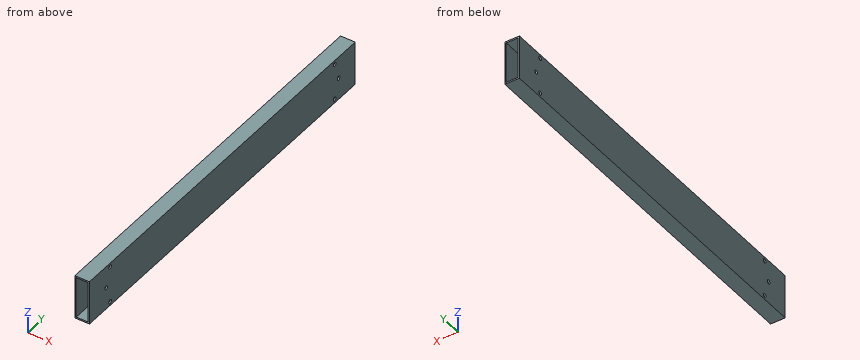
```python
from build123d import *

# Parameters (mm, degrees)
F0_W     = 30
F0_H     = 90
F1_DEPTH = 400
F2_T     = -3
F3_R     = 4
F4_DEPTH = 30.001


# Not quite as in the source:
# - a pattern or mirror of a feature is missing from the dataset's text; its kind, count and spacing are read off the source's solid


with BuildPart() as f1:
    # F0 (on Front) → F1 (new body, symmetric)
    with BuildSketch(Plane.XZ):
        Rectangle(F0_W, F0_H)
    extrude(amount=F1_DEPTH, both=True)

    # F2
    f2_openings = [f1.faces().sort_by_distance(p)[0] for p in [
        (0, -400, 0),
        (0, 400, 0),
    ]]
    offset(amount=F2_T, openings=f2_openings)

    # F3 (on face) → F4 (cut, through all)
    with BuildSketch(Plane.YZ.offset(15)):
        with Locations((338, 37)):
            Circle(F3_R)
        with Locations((350, 0)):
            Circle(F3_R)
        with Locations((338, -37)):
            Circle(F3_R)
    f4 = extrude(amount=-F4_DEPTH, mode=Mode.SUBTRACT)

    # F4_copies: F4 across plane
    add(f4.mirror(Plane(origin=(0, 0, 0), x_dir=(0, 0, -1), z_dir=(0, -1, 0))), mode=Mode.SUBTRACT)


solid = f1.part
```
Here's how the part is built. I have some questions about the finished solid (model axes, mm). Round coordinates to 2 decimals unless told otherwise and drop trailing zeros. Order: outer loops, then holes, each group sorted by start corner. A loop starts at its lowest first (then second) coordinate and runs counter-clockwise, first axis right, second up. Notation, with made-up numbers: M 40.25,3.5 L 46.25,3.5 A13 cw 46.25,28.5 Z; hole C 9,-25 d2. An arc over 180 degrees is marked long. Use CSV: the item, a comma, the result in double quotes.
1) I want a section at C-C (y = 109). List the corners of the cut face in (x, z) for me.
Taken from the geometry:
outline,"M -15,-45 L 15,-45 L 15,45 L -15,45 Z; hole M -12,-42 L 12,-42 L 12,42 L -12,42 Z"
2) I want a section at B-B (x = 1.75). List the corners of the cut face in (y, z) for me, then the cut area to 3 significant figures.
Taken from the geometry:
outline,"M -400,-45 L 400,-45 L 400,-42 L -400,-42 Z; M -400,42 L 400,42 L 400,45 L -400,45 Z"
area,"4,800 mm^2"
3) I need wall thicknesses on line 1 along Z through (x, y) = (-13.5, 338); line 2 along X through (y, z) = (-207.5, -25); line 3 along Z through (x, y) = (13.8, 350). Which ranges of each line are inside material? Lowest first, please. Write a range as [from, to].
Taken from the geometry:
line 1,"[-45, -41], [-33, 33], [41, 45]"
line 2,"[-15, -12], [12, 15]"
line 3,"[-45, -4], [4, 45]"
4) I want a section at A-A (z = -24.5). List the corners of the cut face in (x, y) for me.
Taken from the geometry:
outline,"M -15,-400 L -12,-400 L -12,400 L -15,400 Z; M 12,-400 L 15,-400 L 15,400 L 12,400 Z"
